Geometry check sheet. Reference: the model listing, model coordinates, mm. A direction names the side the tool comes from. Give positions to 0.01 mm unless a question says otherwise; leave off trailing zeros. Order: outer loops, then holes, each group sorted by start corner. A loop starts at its lowest first (then second) coordinate and runs counter-clockwise, first axis right, second up. Notation, with made-up numbers: M 12.25,78.25 L 36.25,78.25 A11 cw 36.25,93.25 Z; hole C 84,52 d8. An arc over 180 degrees is marked long. Answer as CSV lines item,"result". Start each with the question number.
```python
from build123d import *

# Parameters (mm, degrees)
F0_W     = 10
F0_H     = 4.2
F0_W_2   = 4.2
F0_H_2   = 20.833438
F0_H_3   = 4.41329
F1_DEPTH = 4.7


with BuildPart() as f1:
    # F0 (on Top) → F1 (new body)
    with BuildSketch(Plane.XY):
        with BuildLine():
            Line((78.121078, -144.22512), (-60.925064, -144.22512))
            ThreePointArc((-60.925064, -144.22512), (-76.89389, -146.416032), (-90.693977, -154.744361))
            Line((-90.693977, -154.744361), (-105.090827, -167.714982))
            ThreePointArc((-105.090827, -167.714982), (-115.776615, -191.725119), (-105.090827, -215.735257))
            Line((-105.090827, -215.735257), (-90.693977, -228.705877))
            ThreePointArc((-90.693977, -228.705877), (-76.89389, -237.034207), (-60.925064, -239.225119))
            Line((-60.925064, -239.225119), (78.121078, -239.225119))
            ThreePointArc((78.121078, -239.225119), (91.241589, -237.469621), (103.073645, -231.533963))
            ThreePointArc((103.073645, -231.533963), (122.820448, -191.725119), (103.073645, -151.916276))
            ThreePointArc((103.073645, -151.916276), (91.241589, -145.980618), (78.121078, -144.22512))
        make_face()
        with Locations((-37.599309, -191.831764)):
            Rectangle(F0_W, F0_H, mode=Mode.SUBTRACT)
        with Locations((3.80295, -191.725119)):
            Rectangle(F0_W_2, F0_H_2, mode=Mode.SUBTRACT)
        with Locations((48.105208, -191.725119)):
            Rectangle(F0_W_2, F0_H_3, mode=Mode.SUBTRACT)
    extrude(amount=F1_DEPTH)


solid = f1.part
```
Item 1: Section check B-B on x = -75. Record the boundary of the cut face in (y, z).
Item 2: Section check C-C on y = -165.5. Record the boundary of the cut face in (x, z), then the cut area to 3 significant figures.
Item 3: Scan lines: line 1 along X through (y, z) = (-192, 2.95); line 2 along X through (y, z) = (-196.5, 3.1); line 3 along Y through (x, z) = (63.5, 3.2). Record each from-to range of solid material in increasing order.
Item 4: Depth check by flat-ended pin: pin 1 Ø2 at (x, z) = (48.5, 3) entering from -Y; pin 2 Ø1.4 at (x, z) = (-36.5, 2) entering from +Y. Enter the tip coordinate at first touch or a pass-through.
Item 5: Draft check along X on faces 3 (the face through (1.703, -192, 2)), 4 (the face through (5.903, -192, 2)), 5 (the face through (-97.99, -222.13, 2.32)), 6 (the face through (10, -144.225, 2)). Enter one of: pulls with the +X half, pulls with the -X half, needs draft (parallel to the pull), parting line crosses it, or undercut.
Item 6: Section check A-A on z = 2.6. Record the boundary of the cut face in (x, y) (1 decimal).
Item 7: Access from +Z, -Z, +X, -X, +Y, -Y to the whole of each face (thin tool, end or side, straight path). Record for faces 1 (the face through (-38, -193.932, 2)), 2 (the face through (-97.79, -161.14, 2.32)).
Numbers:
1,outline,"M -237.65,0 L -145.8,0 L -145.8,4.7 L -237.65,4.7 Z"
2,outline,"M -102.63,0 L 115.39,0 L 115.39,4.7 L -102.63,4.7 Z"
2,area,"1,020 mm2"
3,line 1,"-115.78 to -42.6, -32.6 to 1.7, 5.9 to 46.01, 50.21 to 122.82"
3,line 2,"-115.42 to 1.7, 5.9 to 122.59"
3,line 3,"-239.23 to -144.23"
4,pin 1,"y = -239.23"
4,pin 2,"y = -144.23"
5,face 3,"undercut"
5,face 4,"undercut"
5,face 5,"pulls with the -X half"
5,face 6,"needs draft"
6,outline,"M -105.1,-215.7 L -90.7,-228.7 A39.9 ccw -60.9,-239.2 L 78.1,-239.2 A40.1 ccw 103.1,-231.5 A50 ccw 103.1,-151.9 A40.1 ccw 78.1,-144.2 L -60.9,-144.2 A39.9 ccw -90.7,-154.7 L -105.1,-167.7 A32.3 ccw Z; hole M -42.6,-193.9 L -32.6,-193.9 L -32.6,-189.7 L -42.6,-189.7 Z; hole M 1.7,-202.1 L 5.9,-202.1 L 5.9,-181.3 L 1.7,-181.3 Z; hole M 46,-193.9 L 50.2,-193.9 L 50.2,-189.5 L 46,-189.5 Z"
7,face 1,"+Z, -Z"
7,face 2,"+Z, -Z, -X, +Y"
